```python
from build123d import *

# Parameters (mm, degrees)
F0_R     = 4.1
F1_DEPTH = 16.25
F0_R_2   = 8.5
F2_DEPTH = 1.5
F4_D     = 6.4


with BuildPart() as f1:
    # F0 (on Top) → F1 (new body)
    with BuildSketch(Plane.XY):
        Circle(F0_R)
    extrude(amount=F1_DEPTH)

    # F0 (on Top) → F2 (join)
    with BuildSketch(Plane.XY):
        Circle(F0_R_2)
        Circle(F0_R, mode=Mode.SUBTRACT)
    extrude(amount=F2_DEPTH)

    # F4 (through all)
    with Locations(Plane(origin=(0, 0, 0), x_dir=(1, 0, 0), z_dir=(0, 0, -1))):
        with Locations((0, 0)):
            Hole(F4_D / 2)


solid = f1.part
```
Here's how the part is built. I have some questions about the finished solid (model axes, mm). Coordinates: 2 decimals unless noted, no trailing zeros. Loops run counter-clockwise (first coordinate to the right, second up) from the corner with the lowest first, then second, coordinate; pieces in that order, holes last. Notation, with made-up numbers: (89.25, 65) - (110.25, 65) arc R13 ccw to (110.25, 82) - close; hole circle Ø2 at (57.25, -22). An arc over 180 degrees is marked (long way). Return JSON: item names as keys, results as strings. Group by question number.
Item 1: We'd pull the mould along X, two halves only. Please class faces 1 (the face through (-0.534, 4.065, 8.772)), 2 (the face through (2.539, 1.947, 8.239)), 3 (the face through (4, 2, 1.5)): +X half, -X half, draft (parallel to the pull), parting line (faces both ways), or undercut.
Item 2: If we section it at C-C on z = 4.5: Write out the boundary of the cut face in (x, y), and give its area (3 significant figures).
Item 3: If we section it at A-A on y = 0: Write out the boundary of the cut face in (x, z).
Item 4: I need wall thicknesses on line 1 (Y direction, x = 0, z = 9.5); line 2 (X direction, y = 2.75, z = 13.75); line 3 (Z direction, x = -6, y = 0.25). Which ranges of each line are inside material? Lowest first, please. Write a range as from..to.
Item 5: Will these pins go through, and if not, where does the flat tip stop? P1, Ø2, axis at y = -1.5, z = 11, coming from the +X side; P2, Ø1, axis at x = -1, y = -1.5, coming from the +Z side; P3, Ø1.5, axis at x = 3, y = 2, coming from the -Z side; P4, Ø4, axis at x = -2, z = 10, coming from the -Y side.
Calculated:
{
 "1": {"face 1": "parting line", "face 2": "undercut", "face 3": "draft"},
 "2": {"outline": "circle Ø8.2 at (0, 0); hole circle Ø6.4 at (0, 0)", "area": "20.6 mm^2"},
 "3": {"outline": "(-8.5, 0) - (-3.2, 0) - (-3.2, 16.25) - (-4.1, 16.25) - (-4.1, 1.5) - (-8.5, 1.5) - close; (3.2, 0) - (8.5, 0) - (8.5, 1.5) - (4.1, 1.5) - (4.1, 16.25) - (3.2, 16.25) - close"},
 "4": {"line 1": "y = -4.1..-3.2, 3.2..4.1", "line 2": "x = -3.04..-1.64, 1.64..3.04", "line 3": "z = 0..1.5"},
 "5": {"P1": "stops at x = 4.07", "P2": "passes through", "P3": "stops at z = 0", "P4": "stops at y = -4.1"}
}
